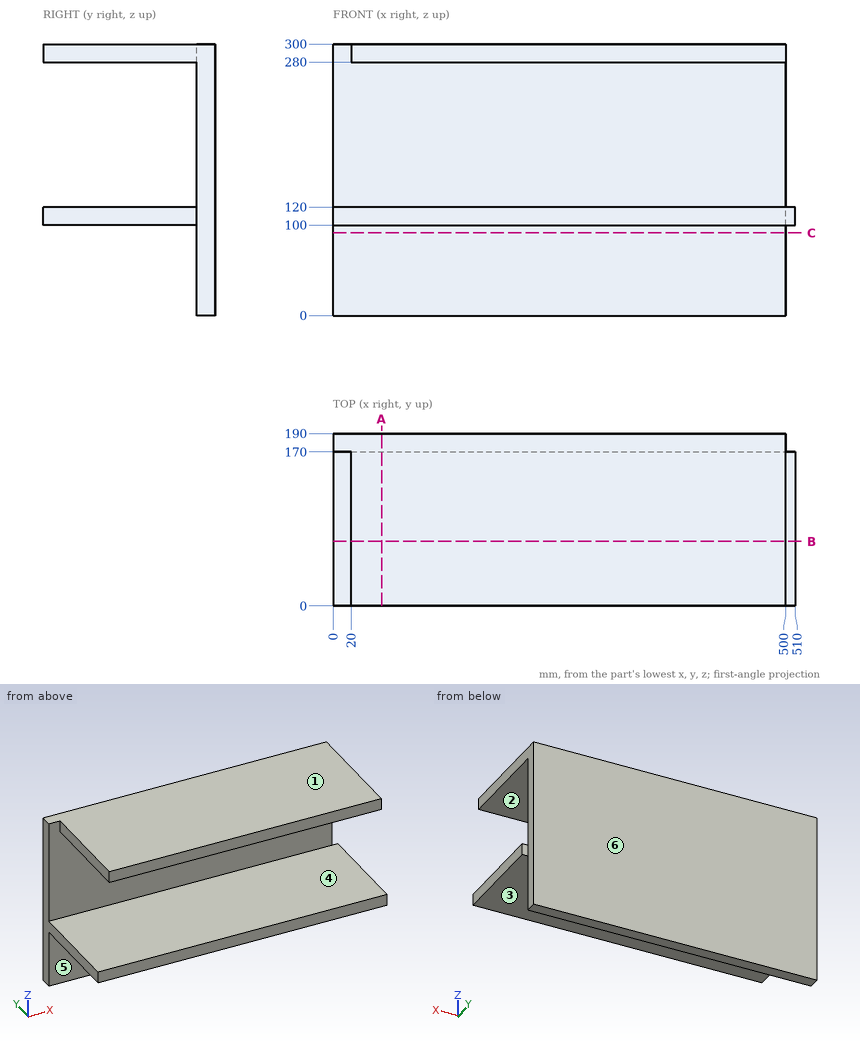
The drawing under review shows one solid part. Ordinate dimensions are in mm from its lowest x, y, z. A direction names the side the tool comes from. Give positions to 0.01 mm unless a question says otherwise; leave off trailing zeros. Loops run counter-clockwise (first coordinate to the right, second up) from the corner with the lowest first, then second, coordinate; pieces in that order, holes last. Notation, with made-up numbers: M -28,-16.75 L 11,-16.75 A25 ccw 11,-3.75 Z; hole C 18,78.5 d3. An arc over 180 degrees is marked long. One line per item, written item: value. Start each with the question number.
Q1. Add section B-B (y = 71). Give the boundary of the cut face in (x, z).
Q2. Machinability: for the marked faces 4, 5 and 6, which of the approach directions +Z, -Z, +X, -X, +Y, -Y give a long, thin tool a straight path to every point of the face, cutting with its end or side? Answer none if there is none.
Q3. Add section C-C (z = 91.5). Give the boundary of the cut face in (x, y), and give its area (3 significant figures).
Q4. Add section A-A (x = 53.5). Give the boundary of the cut face in (y, z).
Q5. Draft analysis for pull direction Z (two halves, no side actions). For the marked faces 1, 2 and 3, state which applies: released by +Z, released by -Z, zero draft, split by the parting line, or undercut.
Q6. Clearance check with flat-ended pins moving along their axes: pin 1 Ø10 at (y, z) = (124.5, 291) entering from -X; pin 2 Ø12 at (x, y) = (437, 143) entering from -Z; pin 3 Ø1.5 at (x, z) = (119.5, 175) entering from -Y. State where each tip first meets the part, or that it passes through.
Q7. For L1, parallel to Z at x = 432, y = 66.5; L2, parallel to Y at x = 407.5, z = 188, list the stretches that pass through material, from the lowest coordinate up.
Reply:
1. outline: M 0,100 L 510,100 L 510,120 L 0,120 Z; M 20,280 L 500,280 L 500,300 L 20,300 Z
2. face 4: +X, -X, -Y
2. face 5: -Z, +X, -X, -Y
2. face 6: +Z, -Z, +X, -X, +Y
3. outline: M 0,170 L 500,170 L 500,190 L 0,190 Z
3. area: 10,000 mm²
4. outline: M 0,100 L 170,100 L 170,0 L 190,0 L 190,300 L 0,300 L 0,280 L 170,280 L 170,120 L 0,120 Z
5. face 1: released by +Z
5. face 2: undercut
5. face 3: released by -Z
6. pin 1: x = 20
6. pin 2: z = 100
6. pin 3: y = 170
7. L1: 100 to 120, 280 to 300
7. L2: 170 to 190
